from build123d import *

# Parameters (mm, degrees)
SKETCH_6_W          = 122.5
SKETCH_6_H          = 122.5
EXTRUDE_5_DEPTH     = 160
SKETCH_7_R          = 17.5
EXTRUDE_6_DEPTH     = 55.5
SKETCH_8_R          = 6
EXTRUDE_7_DEPTH     = 5
CHAMFER_1_SIZE      = 5
SKETCH_9_R          = 2.75
CUT_EXTRUDE_1_DEPTH = 20


with BuildPart() as part:
    # 草图6 → 凸台-拉伸5 (new body)
    with BuildSketch(Plane.XY):
        Rectangle(SKETCH_6_W, SKETCH_6_H)
    extrude(amount=EXTRUDE_5_DEPTH)

    # 草图7 → 凸台-拉伸6 (add)
    with BuildSketch(Plane.XZ.offset(61.25)):
        with Locations(Location((0, 25, 0), (0, 0, 90))):
            Circle(SKETCH_7_R)
    extrude(amount=EXTRUDE_6_DEPTH)

    # 草图8 → 凸台-拉伸7 (add)
    with BuildSketch(Plane.XZ.offset(116.75)):
        with Locations(Location((0, 25, 0), (0, 0, 270))):
            Circle(SKETCH_8_R)
    extrude(amount=EXTRUDE_7_DEPTH)

    # 倒角1
    chamfer_1_edges = [part.edges().sort_by_distance(p)[0] for p in [
        (-61.25, 61.25, 80),
        (61.25, 61.25, 80),
        (61.25, -61.25, 80),
        (-61.25, -61.25, 80),
    ]]
    chamfer(chamfer_1_edges, length=CHAMFER_1_SIZE)

    # 草图9 → 切除-拉伸1 (cut)
    with BuildSketch(Plane(origin=(0, 0, 0), x_dir=(-1, 0, 0), z_dir=(0, 0, -1))):
        with Locations((-48, 48)):
            Circle(SKETCH_9_R)
        with Locations((48, 48)):
            Circle(SKETCH_9_R)
        with Locations((48, -48)):
            Circle(SKETCH_9_R)
        with Locations((-48, -48)):
            Circle(SKETCH_9_R)
    extrude(amount=-CUT_EXTRUDE_1_DEPTH, mode=Mode.SUBTRACT)


solid = part.part
Verification items for the finished model (mm, model axes). A direction names the side the tool comes from. Coordinates: 2 decimals unless noted, no trailing zeros. Write each loop counter-clockwise with the first axis right and the second up, starting at its lowest first coordinate (ties: lowest second). Pieces come first, ordered by that corner, then holes. Notation, with made-up numbers: M -30.5,13 L -9.5,13 A20 cw -9.5,46 Z; hole C -40,33.25 d10. An arc over 180 degrees is marked long. Use CSV: the item, a comma, the result in double quotes.
Q1. Section check C-C, the plane y = -86. Enter the section's corners in (x, z), and give its area (3 significant figures).
Computed values:
outline,"C 0,25 d35"
area,"962 mm²"
Q2. Section check D-D, the plane z = 25. Enter the section's corners in (x, y), and give its area (3 significant figures).
Computed values:
outline,"M -61.25,-56.25 L -56.25,-61.25 L -17.5,-61.25 L -17.5,-116.75 L -6,-116.75 L -6,-121.75 L 6,-121.75 L 6,-116.75 L 17.5,-116.75 L 17.5,-61.25 L 56.25,-61.25 L 61.25,-56.25 L 61.25,56.25 L 56.25,61.25 L -56.25,61.25 L -61.25,56.25 Z"
area,"17,000 mm²"
Q3. Section check B-B, the plane x = -48. Enter the section's corners in (y, z), and give its area (3 significant figures).
Computed values:
outline,"M -61.25,0 L -50.75,0 L -50.75,20 L -45.25,20 L -45.25,0 L 45.25,0 L 45.25,20 L 50.75,20 L 50.75,0 L 61.25,0 L 61.25,160 L -61.25,160 Z"
area,"19,400 mm²"
Q4. Thickness scan on line 1 along Y through (x, z) = (48, 9); line 2 along Y through (x, z) = (0, 9.5); line 3 along Y through (x, z) = (48.5, 86). Record the ranges inside material, lowest first. Write a range as [from, to].
Computed values:
line 1,"[-61.25, -50.75], [-45.25, 45.25], [50.75, 61.25]"
line 2,"[-116.75, 61.25]"
line 3,"[-61.25, 61.25]"
Q5. Section check A-A, the plane z = 145. Enter the section's corners in (x, y), and give its area (3 significant figures).
Computed values:
outline,"M -61.25,-56.25 L -56.25,-61.25 L 56.25,-61.25 L 61.25,-56.25 L 61.25,56.25 L 56.25,61.25 L -56.25,61.25 L -61.25,56.25 Z"
area,"15,000 mm²"
Q6. Set-up check for faces 4 (the cylindrical face through (0, -119, 31)), 5 (the flat face through (0, -121.75, 25)), 6 (the flat face through (-48, -48, 20)): record each of +Z, -Z, +X, -X, +Y, -Y from which the full face is reachable in a straight line by a thin tool's end or side.
Computed values:
face 4,"-Y"
face 5,"+Z, -Z, +X, -X, -Y"
face 6,"-Z"
Q7. Mould release check, pull along X, two halves, no side actions. Record for faces 1 (the flat face through (0, -116.75, 33)), 2 (the flat face through (48, -48, 20)), 3 (the flat face through (-61.25, -1, 79)): pulls with the +X half, pulls with the -X half, needs draft (parallel to the pull), parting line crosses it, or undercut.
Computed values:
face 1,"needs draft"
face 2,"undercut"
face 3,"pulls with the -X half"
Q8. Go/stop test with flat-tipped pins: P1, Ø4.5, axis at x = -48, y = -48, coming from the -Z side; P2, Ø5, axis at x = 42, z = 42, coming from the -Y side; P3, Ø5, axis at x = 15, y = -97, coming from the -Z side. Record where each tip stops, or that it passes through.
Computed values:
P1,"z = 20"
P2,"y = -61.25"
P3,"z = 12.75"
